```python
from build123d import *

# Parameters (mm, degrees)
BOSS_EXTRUDE1_DEPTH = 4.7625
SKETCH2_W           = 80
SKETCH2_H           = 2.5
CUT_EXTRUDE1_DEPTH  = 4.7625
BOSS_EXTRUDE2_DEPTH = 9.525


with BuildPart() as part:
    # Sketch1 → Boss-Extrude1 (new, symmetric)
    with BuildSketch(Plane.XY):
        with BuildLine():
            Line((-790, 21.9056), (790, 21.9056))
            ThreePointArc((790, 21.9056), (811.9056, 0), (790, -21.9056))
            Line((790, -21.9056), (-790, -21.9056))
            ThreePointArc((-790, -21.9056), (-811.9056, 0), (-790, 21.9056))
        make_face()
        with BuildLine():
            Line((-790, -19.4056), (790, -19.4056))
            ThreePointArc((790, -19.4056), (809.4056, 0), (790, 19.4056))
            Line((790, 19.4056), (-790, 19.4056))
            ThreePointArc((-790, 19.4056), (-809.4056, 0), (-790, -19.4056))
        make_face(mode=Mode.SUBTRACT)
    extrude(amount=BOSS_EXTRUDE1_DEPTH, both=True)

    # Sketch2 → Cut-Extrude1 (cut, symmetric)
    with BuildSketch(Plane.XY):
        with Locations((0, 20.6556)):
            Rectangle(SKETCH2_W, SKETCH2_H)
    extrude(amount=CUT_EXTRUDE1_DEPTH, both=True, mode=Mode.SUBTRACT)

    # Sketch3 → Boss-Extrude2 (add)
    with BuildSketch(Plane.XY.offset(4.7625)):
        Polygon((-41.25, 21.9056), (-38.75, 21.9056), (-38.75, 11.9056), (-53.25, 11.9056), (-53.25, 14.4056), (-41.25, 14.4056), align=None)
        Polygon((53.25, 11.9056), (38.75, 11.9056), (38.75, 21.9056), (41.25, 21.9056), (41.25, 14.4056), (53.25, 14.4056), align=None)
    extrude(amount=-BOSS_EXTRUDE2_DEPTH)


solid = part.part
```
The model under review builds one solid part; all positions refer to its coordinate system, in mm. Round coordinates to 2 decimals unless told otherwise and drop trailing zeros. Write each loop counter-clockwise with the first axis right and the second up, starting at its lowest first coordinate (ties: lowest second). Pieces come first, ordered by that corner, then holes. Notation, with made-up numbers: M 10.5,-2.75 L 53.5,-2.75 A22 ccw 53.5,36.25 Z; hole C -20.5,49 d6. An arc over 180 degrees is marked long. Use CSV: the item, a comma, the result in double quotes. Start each with the question number.
(1) Clearance check with flat-ended pins moving along their axes: P1, Ø3, axis at y = 15, z = -0.5, coming from the +X side; P2, Ø3, axis at y = -7, z = -2.5, coming from the +X side; P3, Ø0.8, axis at y = 12.5, z = 1.5, coming from the +X side. State where each tip first meets the part, or that it passes through.
(2) We need section A-A, the plane y = 0. State the section outline as (x, z) points.
(3) We need section B-B, the plane x = 233. State the section outline as (y, z) points, then the cut area to 3 significant figures.
(4) For line 1 along Y through (x, z) = (204.5, 4); line 2 along X through (y, z) = (1.5, -2.25); line 3 along Y through (x, z) = (48.5, -1.5), list the stretches that pass through material, from the lowest coordinate up.
(5) We need section C-C, the plane z = -0.75. State the section outline as (x, y) points.
Findings:
1,P1,"x = 807.25"
1,P2,"x = 811.2"
1,P3,"x = 808.26"
2,outline,"M -811.91,-4.76 L -809.41,-4.76 L -809.41,4.76 L -811.91,4.76 Z; M 809.41,-4.76 L 811.91,-4.76 L 811.91,4.76 L 809.41,4.76 Z"
3,outline,"M -21.91,-4.76 L -19.41,-4.76 L -19.41,4.76 L -21.91,4.76 Z; M 19.41,-4.76 L 21.91,-4.76 L 21.91,4.76 L 19.41,4.76 Z"
3,area,"47.6 mm^2"
4,line 1,"-21.91 to -19.41, 19.41 to 21.91"
4,line 2,"-811.85 to -809.35, 809.35 to 811.85"
4,line 3,"-21.91 to -19.41, 11.91 to 14.41, 19.41 to 21.91"
5,outline,"M -790,-21.91 L 790,-21.91 A21.91 ccw 790,21.91 L 38.75,21.91 L 38.75,11.91 L 53.25,11.91 L 53.25,14.41 L 41.25,14.41 L 41.25,19.41 L 790,19.41 A19.41 cw 790,-19.41 L -790,-19.41 A19.41 cw -790,19.41 L -41.25,19.41 L -41.25,14.41 L -53.25,14.41 L -53.25,11.91 L -38.75,11.91 L -38.75,21.91 L -790,21.91 A21.91 ccw Z"
